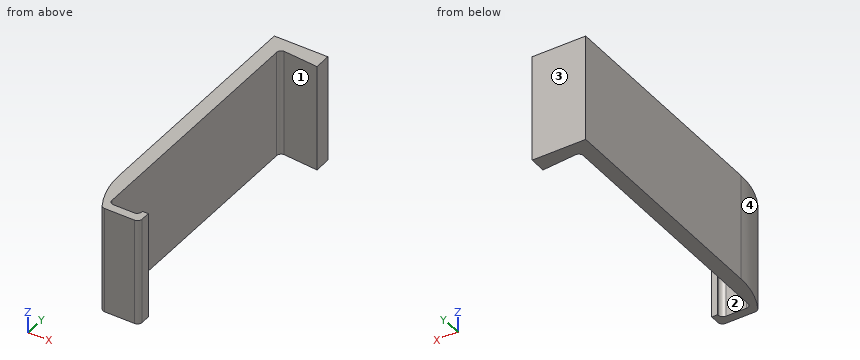
from build123d import *

# Parameters (mm, degrees)
F1_DEPTH = 30


# Not quite as in the source:
# - a feature names something its author has since deleted; it is built from what else it names


with BuildPart() as f1:
    # F0 (on Top) → F1 (new body)
    with BuildSketch(Plane.XY):
        with BuildLine():
            Line((15.0259537622, 74.3470937014), (15, 79))
            Line((15, 79), (0, 79))
            Line((0, 79), (0, 12.7))
            ThreePointArc((0, 12.7), (0.8280772268, 6.4500404007), (3.2551662494, 0.6313682358))
            ThreePointArc((3.2551662494, 0.6313682358), (3.719732188, 0.1690998364), (4.352913702, 0))
            Line((4.352913702, 0), (12.7432, 0))
            ThreePointArc((12.7432, 0), (13.6412256121, 0.3719743879), (14.0132, 1.27))
            Line((14.0132, 1.27), (14.0132, 3.9116))
            Line((14.0132, 3.9116), (12.3622, 3.9116))
            Line((12.3622, 3.9116), (12.3622, 3.6322))
            ThreePointArc((12.3622, 3.6322), (11.9902256121, 2.7341743879), (11.0922, 2.3622))
            Line((11.0922, 2.3622), (5.2832, 2.3622))
            ThreePointArc((5.2832, 2.3622), (4.3851743879, 2.7341743879), (4.0132, 3.6322))
            Line((4.0132, 3.6322), (4.0132, 73.92))
            ThreePointArc((4.0132, 73.92), (4.3851743879, 74.8180256121), (5.2832, 75.19))
            Line((5.2832, 75.19), (15.0259537622, 74.3470937014))
        make_face()
    extrude(amount=F1_DEPTH)


solid = f1.part
For this review, take the finished solid that the model builds, in its own axes (mm). Face numbers are marked on the shaded views. Give positions to 0.01 mm unless a question says otherwise; leave off trailing zeros. Order: outer loops, then holes, each group sorted by start corner. A loop starts at its lowest first (then second) coordinate and runs counter-clockwise, first axis right, second up. Notation, with made-up numbers: (88, 10.5) - (120, 10.5) arc R24 ccw to (120, 39.5) - close; hole circle Ø1 at (23.5, 29.5). An arc over 180 degrees is marked (long way). Answer as a JSON object with one key per item and string values. Group by question number.
Item 1: Draft analysis for pull direction X (two halves, no side actions). For the marked faces 1, 2, 3 and 4, state which applies: pulls with the +X half, pulls with the -X half, needs draft (parallel to the pull), parting line crosses it, or undercut.
Item 2: Take a section at B-B on x = 8.25. Give the boundary of the cut face in (y, z), and give its area (3 significant figures).
Item 3: Take a section at C-C on y = 55. Give the boundary of the cut face in (x, z).
Item 4: Take a section at A-A on z = 3. Give the boundary of the cut face in (x, y).
Item 5: Take a section at D-D on y = 7. Give the boundary of the cut face in (x, z), and give its area (3 significant figures).
Item 6: Clearance check with flat-ended pins moving along their axes: pin 1 Ø3 at (y, z) = (2, 22) entering from +X; pin 2 Ø9 at (y, z) = (36.5, 20) entering from +X. State where each tip first meets the part, or that it passes through.
Item 7: Wall thickness on line 1 along X through (y, z) = (19.5, 14.25); line 2 along Y through (x, z) = (5.75, 17); line 3 along Y through (x, z) = (11.75, 6): over which ranges is each line inside the solid? List them lowest first.
Reported:
{
 "1": {"face 1": "undercut", "face 2": "undercut", "face 3": "needs draft", "face 4": "pulls with the -X half"},
 "2": {"outline": "(0, 0) - (2.36, 0) - (2.36, 30) - (0, 30) - close; (74.93, 0) - (79, 0) - (79, 30) - (74.93, 30) - close", "area": "193 mm^2"},
 "3": {"outline": "(0, 0) - (4.01, 0) - (4.01, 30) - (0, 30) - close"},
 "4": {"outline": "(0, 12.7) arc R24 ccw to (3.26, 0.63) arc R1.27 ccw to (4.35, 0) - (12.74, 0) arc R1.27 ccw to (14.01, 1.27) - (14.01, 3.91) - (12.36, 3.91) - (12.36, 3.63) arc R1.27 cw to (11.09, 2.36) - (5.28, 2.36) arc R1.27 cw to (4.01, 3.63) - (4.01, 73.92) arc R1.27 cw to (5.28, 75.19) - (15.03, 74.35) - (15, 79) - (0, 79) - close"},
 "5": {"outline": "(0.69, 0) - (4.01, 0) - (4.01, 30) - (0.69, 30) - close", "area": "99.8 mm^2"},
 "6": {"pin 1": "x = 14.01", "pin 2": "x = 4.01"},
 "7": {"line 1": "0 to 4.01", "line 2": "0 to 2.36, 75.15 to 79", "line 3": "0 to 2.55, 74.63 to 79"}
}
